Verification items for the finished model (mm, model axes). Give positions to 0.01 mm unless a question says otherwise; leave off trailing zeros. Order: outer loops, then holes, each group sorted by start corner. A loop starts at its lowest first (then second) coordinate and runs counter-clockwise, first axis right, second up. Notation, with made-up numbers: (67, 74) - (107, 74) arc R21 ccw to (107, 108) - close; hole circle Ø1 at (-18.75, 0). An arc over 180 degrees is marked (long way). Answer as a JSON object with one key per item and string values. Group by question number.
(1) Section check B-B (y = 0). Record the boundary of the cut face in (x, z).
(2) Section check A-A (x = -1.5). Record the boundary of the cut face in (y, z).
(3) Thickness scan on line 1 (Z direction, x = -5, y = -5.25); line 2 (X direction, y = -0.25, z = -0.5). Record the ranges inside material, lowest first.
(4) Section check D-D (y = -3.75). Record the boundary of the cut face in (x, z).
```python
from build123d import *

# Parameters (mm, degrees)
F0_W     = 13
F0_H     = 13
F1_DEPTH = 14
F2_R     = 1
F3_DEPTH = 1
F4_R     = 2
F5_DEPTH = 1.2


with BuildPart() as f1:
    # F0 (on Top) → F1 (new body)
    with BuildSketch(Plane.XY):
        Rectangle(F0_W, F0_H)
    extrude(amount=F1_DEPTH)

    # F2 (on face) → F3 (join)
    with BuildSketch(Plane(origin=(0, 0, 0), x_dir=(1, 0, 0), z_dir=(0, 0, -1))):
        Circle(F2_R)
    extrude(amount=F3_DEPTH)

    # F4 (on face) → F5 (join)
    with BuildSketch(Plane(origin=(0, 0, -1), x_dir=(1, 0, 0), z_dir=(0, 0, -1))):
        Circle(F4_R)
    extrude(amount=F5_DEPTH)


solid = f1.part
```
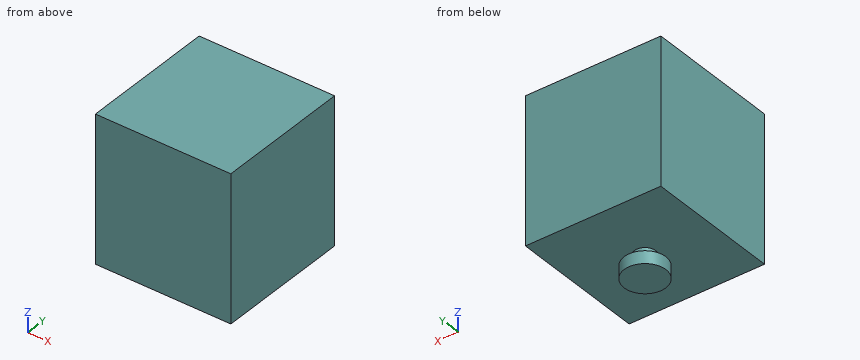
Solutions:
{
 "1": {"outline": "(-6.5, 0) - (-1, 0) - (-1, -1) - (-2, -1) - (-2, -2.2) - (2, -2.2) - (2, -1) - (1, -1) - (1, 0) - (6.5, 0) - (6.5, 14) - (-6.5, 14) - close"},
 "2": {"outline": "(-6.5, 0) - (6.5, 0) - (6.5, 14) - (-6.5, 14) - close; (-1.32, -2.2) - (1.32, -2.2) - (1.32, -1) - (-1.32, -1) - close"},
 "3": {"line 1": "z = 0 to 14", "line 2": "x = -0.97 to 0.97"},
 "4": {"outline": "(-6.5, 0) - (6.5, 0) - (6.5, 14) - (-6.5, 14) - close"}
}
